from build123d import *

# Parameters (mm, degrees)
SKETCH1_W           = 404
SKETCH1_H           = 132
BOSS_EXTRUDE1_DEPTH = 3


with BuildPart() as part:
    # Sketch1 → Boss-Extrude1 (new body)
    with BuildSketch(Plane.XY.offset(152)):
        with Locations((85.526581968, -69.40919868)):
            Rectangle(SKETCH1_W, SKETCH1_H)
        with BuildLine():
            Line((-96.473418032, -105.888993971), (-96.473418032, -29.929403389))
            ThreePointArc((-96.473418032, -29.929403389), (-94.516026587, -25.961717264), (-90.176404758, -25.100557091))
            Line((-90.176404758, -25.100557091), (51.22430223, -63.080352382))
            ThreePointArc((51.22430223, -63.080352382), (54.927288957, -67.90919868), (51.22430223, -72.738044978))
            Line((51.22430223, -72.738044978), (-90.176404758, -110.717840269))
            ThreePointArc((-90.176404758, -110.717840269), (-94.516026587, -109.856680096), (-96.473418032, -105.888993971))
        make_face(mode=Mode.SUBTRACT)
        with BuildLine():
            Line((152.536061434, -23.40919868), (18.517102502, -23.40919868))
            ThreePointArc((18.517102502, -23.40919868), (13.560075596, -27.755070057), (17.220089228, -33.238044978))
            Line((17.220089228, -33.238044978), (84.229568694, -51.236585203))
            ThreePointArc((84.229568694, -51.236585203), (85.526581968, -51.407738905), (86.823595242, -51.236585203))
            Line((86.823595242, -51.236585203), (153.833074707, -33.238044978))
            ThreePointArc((153.833074707, -33.238044978), (157.493088339, -27.755070057), (152.536061434, -23.40919868))
        make_face(mode=Mode.SUBTRACT)
        with BuildLine():
            Line((261.229568694, -25.100557091), (119.828861705, -63.080352382))
            ThreePointArc((119.828861705, -63.080352382), (116.125874979, -67.90919868), (119.828861705, -72.738044978))
            Line((119.828861705, -72.738044978), (261.229568694, -110.717840269))
            ThreePointArc((261.229568694, -110.717840269), (265.569190522, -109.856680096), (267.526581968, -105.888993971))
            Line((267.526581968, -105.888993971), (267.526581968, -29.929403389))
            ThreePointArc((267.526581968, -29.929403389), (265.569190522, -25.961717264), (261.229568694, -25.100557091))
        make_face(mode=Mode.SUBTRACT)
        with BuildLine():
            Line((17.220089228, -102.580352382), (84.229568694, -84.581812156))
            ThreePointArc((84.229568694, -84.581812156), (85.526581968, -84.410658454), (86.823595242, -84.581812156))
            Line((86.823595242, -84.581812156), (153.833074707, -102.580352382))
            ThreePointArc((153.833074707, -102.580352382), (157.493088339, -108.063327303), (152.536061434, -112.40919868))
            Line((152.536061434, -112.40919868), (18.517102502, -112.40919868))
            ThreePointArc((18.517102502, -112.40919868), (13.560075596, -108.063327303), (17.220089228, -102.580352382))
        make_face(mode=Mode.SUBTRACT)
    extrude(amount=BOSS_EXTRUDE1_DEPTH)


solid = part.part
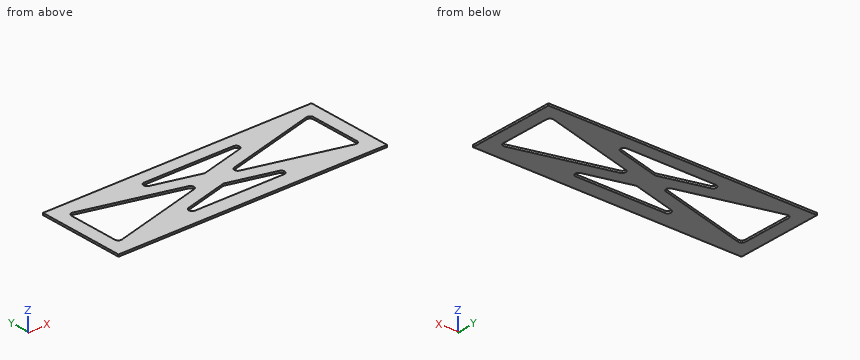
Design review of the part built by this model. Coordinates are the model's own, in mm. Coordinates: 2 decimals unless noted, no trailing zeros. Loops run counter-clockwise (first coordinate to the right, second up) from the corner with the lowest first, then second, coordinate; pieces in that order, holes last.
Item 1: Add section D-D (x = -66). Write out the cut boundary in (y, z), and give its area (3 significant figures).
Completed:
outline: (-135.41, 152) - (-104.22, 152) - (-104.22, 155) - (-135.41, 155) - close; (-31.59, 152) - (-3.41, 152) - (-3.41, 155) - (-31.59, 155) - close
area: 178 mm2
Item 2: Add section C-C (y = -57.5). Write out the cut boundary in (x, z), and give its area (3 significant figures).
Completed:
outline: (-116.47, 152) - (-96.47, 152) - (-96.47, 155) - (-116.47, 155) - close; (30.45, 152) - (140.6, 152) - (140.6, 155) - (30.45, 155) - close; (267.53, 152) - (287.53, 152) - (287.53, 155) - (267.53, 155) - close
area: 450 mm2
Item 3: Add section B-B (x = 70). Write out the cut boundary in (y, z).
Completed:
outline: (-135.41, 152) - (-112.41, 152) - (-112.41, 155) - (-135.41, 155) - close; (-88.4, 152) - (-47.41, 152) - (-47.41, 155) - (-88.4, 155) - close; (-23.41, 152) - (-3.41, 152) - (-3.41, 155) - (-23.41, 155) - close
Item 4: Add section A-A (z = 153.2). Write out the cut boundary in (x, y).
Completed:
outline: (-116.47, -135.41) - (287.53, -135.41) - (287.53, -3.41) - (-116.47, -3.41) - close; hole (-96.47, -105.89) arc R5 ccw to (-90.18, -110.72) - (51.22, -72.74) arc R5 ccw to (51.22, -63.08) - (-90.18, -25.1) arc R5 ccw to (-96.47, -29.93) - close; hole (17.22, -102.58) arc R5 ccw to (18.52, -112.41) - (152.54, -112.41) arc R5 ccw to (153.83, -102.58) - (86.82, -84.58) arc R5 ccw to (84.23, -84.58) - close; hole (17.22, -33.24) - (84.23, -51.24) arc R5 ccw to (86.82, -51.24) - (153.83, -33.24) arc R5 ccw to (152.54, -23.41) - (18.52, -23.41) arc R5 ccw to start; hole (119.83, -72.74) - (261.23, -110.72) arc R5 ccw to (267.53, -105.89) - (267.53, -29.93) arc R5 ccw to (261.23, -25.1) - (119.83, -63.08) arc R5 ccw to start
Item 5: Wall thickness on L1, parallel to Y at x = 74, z = 153.2; L2, parallel to Y at x = 131, z = 153.45; L3, parallel to Y at x = -90, z = 153.35: over which ranges is each line inside the solid? List them lowest first.
Completed:
L1: y = -135.41 to -112.41, -87.33 to -48.49, -23.41 to -3.41
L2: y = -135.41 to -112.41, -96.45 to -75.74, -60.08 to -39.37, -23.41 to -3.41
L3: y = -135.41 to -110.67, -25.15 to -3.41
